Part model, mm, in its own coordinate system. A direction names the side the tool comes from. Give positions to 0.01 mm unless a question says otherwise; leave off trailing zeros. Loops run counter-clockwise (first coordinate to the right, second up) from the corner with the lowest first, then second, coordinate; pieces in that order, holes last. Notation, with made-up numbers: M 18,59.5 L 52,59.5 A18 ccw 52,94.5 Z; hole C 38,11.25 d8. An arc over 180 degrees is marked long. Put each result on its own line as item: value. Start each with the question number.
```python
from build123d import *

# Parameters (mm, degrees)
SKETCH1_W                = 45.5
SKETCH1_H                = 20.2
BOSS_EXTRUDE1_DEPTH      = 3
SKETCH2_R                = 8
BOSS_EXTRUDE2_DEPTH      = 13.8
SKETCH3_W                = 10.5
SKETCH3_H                = 4.5
BOSS_EXTRUDE3_DEPTH      = 4
FILLET1_R                = 2.25
BOSS_EXTRUDE4_DEPTH      = 10
BOSS_EXTRUDE4_DEPTH_BACK = 5
SKETCH4_W                = 10.16
SKETCH4_H                = 2.54


with BuildPart() as part:
    # Sketch1 → Boss-Extrude1 (new body)
    with BuildSketch(Plane.XY):
        Rectangle(SKETCH1_W, SKETCH1_H)
    extrude(amount=BOSS_EXTRUDE1_DEPTH)

    # Sketch2 → Boss-Extrude2 (add)
    with BuildSketch(Plane.XY.offset(3)):
        with Locations(Location((-13.5, 0, 0), (0, 0, 180))):
            Circle(SKETCH2_R)
        with Locations(Location((13.5, 0, 0), (0, 0, 180))):
            Circle(SKETCH2_R)
    extrude(amount=BOSS_EXTRUDE2_DEPTH)

    # Sketch3 → Boss-Extrude3 (add)
    with BuildSketch(Plane.XY.offset(3)):
        with Locations((0, 7.35)):
            Rectangle(SKETCH3_W, SKETCH3_H)
    extrude(amount=BOSS_EXTRUDE3_DEPTH)

    # Fillet1
    fillet1_edges = [part.edges().sort_by_distance(p)[0] for p in [
        (-5.25, 5.1, 5),
        (-5.25, 9.6, 5),
        (5.25, 5.1, 5),
        (5.25, 9.6, 5),
    ]]
    fillet(fillet1_edges, radius=FILLET1_R - 0.0001)  # a hair under: the kernel refuses the full size

    # Sketch4 → Boss-Extrude4 (add, two sides: drawn at the far end of the back side and taken through both)
    with BuildSketch(Plane(origin=(0, 0, 0), x_dir=(-1, 0, 0), z_dir=(0, 0, -1)).offset(-BOSS_EXTRUDE4_DEPTH_BACK)):
        with Locations((0, -8.83)):
            Rectangle(SKETCH4_W, SKETCH4_H)
    extrude(amount=BOSS_EXTRUDE4_DEPTH + BOSS_EXTRUDE4_DEPTH_BACK)


solid = part.part
```
1) Pin check, flat tips, straight feed: pin 1 Ø2 at (x, y) = (1.5, 7.5) entering from +Z; pin 2 Ø1.6 at (y, z) = (-9, 4) entering from +X; pin 3 Ø1.6 at (y, z) = (-9, 4) entering from -X; pin 4 Ø12 at (x, z) = (-18, -4) entering from -Y. Stop position of each tip, or through.
2) Which spindle directions (+Z, -Z, +X, -X, +Y, -Y) get a long thin tool onto all of the face, cutting with end or side? Do faces 4 (the cylindrical face through (4.61, 8.92, 5.03)), 5 (the cylindrical face through (4.57, 5.74, 5.03)), 6 (the flat face through (0, -7.56, -5)), 7 (the flat face through (5.08, -9, -5)). Say none if no direction does.
3) Band-saw the part on B-B on x = -1.5. Give the cut face in (y, z), then the cut area to 3 significant figures.
4) Band-saw the part on C-C on y = 0. Give the cut face in (x, z), then the cut area to 3 significant figures.
5) Band-saw the part on A-A on z = 3.75. State how many separate pieces and enclosed holes the cut face has, then the cut area to 3 significant figures.
6) Band-saw the part on D-D on z = 7.75. Give the cut face in (x, y), then the cut area to 3 significant figures.
7) Mould opens along Y. For faces 1 (the flat face through (0, -7.56, 4)), 2 (the cylindrical face through (15.23, 7.81, 9.8)), 3 (the flat face through (-13, 0, 16.8)) say: +Y half, -Y half, draft (parallel to the pull), parting line (faces both ways), or undercut.
8) Wall check: L1, parallel to X at y = 0.25, z = 15.75; L2, parallel to Z at x = 20.5, y = -3; L3, parallel to Z at x = 3, y = 8.5. Give the ranges that are in metal, low to high.
Evaluation:
1. pin 1: z = 7
1. pin 2: x = 5.08
1. pin 3: x = -5.08
1. pin 4: y = -10.1
2. face 4: +Z, +Y
2. face 5: +Z
2. face 6: -Z, +X, -X, +Y
2. face 7: -Z, +X, +Y, -Y
3. outline: M -10.1,-10 L -7.56,-10 L -7.56,0 L 10.1,0 L 10.1,3 L 9.6,3 L 9.6,7 L 5.1,7 L 5.1,3 L -7.56,3 L -7.56,5 L -10.1,5 Z
3. area: 109 mm2
4. outline: M -22.75,0 L 22.75,0 L 22.75,3 L 21.5,3 L 21.5,16.8 L 5.5,16.8 L 5.5,3 L -5.5,3 L -5.5,16.8 L -21.5,16.8 L -21.5,3 L -22.75,3 Z
4. area: 578 mm2
5. separate pieces: 4
5. enclosed holes: 0
5. area: 471 mm2
6. outline: C -13.5,0 d16; C 13.5,0 d16
6. area: 402 mm2
7. face 1: undercut
7. face 2: parting line
7. face 3: draft
8. L1: -21.5 to -5.5, 5.5 to 21.5
8. L2: 0 to 16.8
8. L3: 0 to 7
